CAD build for the part. Positions are in the model's coordinates, mm. Face numbers are marked on the shaded views. A direction names the side the tool comes from. Give positions to 0.01 mm unless a question says otherwise; leave off trailing zeros. Loops run counter-clockwise (first coordinate to the right, second up) from the corner with the lowest first, then second, coordinate; pieces in that order, holes last. Notation, with made-up numbers: M 64,-3.5 L 83,-3.5 A6 ccw 83,4.5 Z; hole C 47,-13 d10. An arc over 180 degrees is marked long. Answer as CSV lines item,"result".
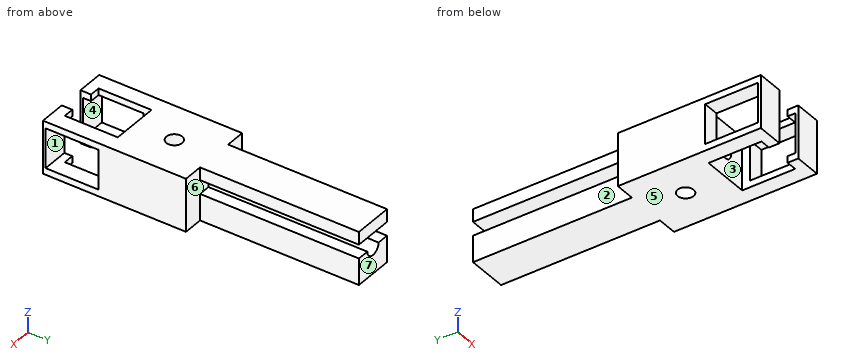
from build123d import *

# Parameters (mm, degrees)
F0_R     = 3.81
F0_W     = 7.62
F0_H     = 25.4
F0_H_2   = 5.08
F0_W_2   = 5.08
F1_DEPTH = 25.4
F2_R     = 3.81
F3_DEPTH = 114.301
F4_W     = 25.4
F4_H     = 19.05
F5_DEPTH = 38.101
F6_W     = 76.2
F6_H     = 6.593191
F7_DEPTH = 28.576


with BuildPart() as f1:
    # F0 (on Top) → F1 (new body)
    with BuildSketch(Plane.XY):
        Polygon((-9.525, 19.05), (-19.05, 19.05), (-19.05, -19.05), (-11.43, -19.05), (11.43, -19.05), (19.05, -19.05), (19.05, 19.05), (9.525, 19.05), (0, 19.05), align=None)
        Circle(F0_R, mode=Mode.SUBTRACT)
        Polygon((-9.525, 95.25), (-9.525, 19.05), (0, 19.05), (9.525, 19.05), (9.525, 95.25), align=None)
        with Locations((-15.24, -31.75)):
            Rectangle(F0_W, F0_H)
        with Locations((-15.24, -46.99)):
            Rectangle(F0_W, F0_H_2)
        with Locations((15.24, -31.75)):
            Rectangle(F0_W, F0_H)
        with Locations((-8.89, -46.99)):
            Rectangle(F0_W_2, F0_H_2)
        with Locations((15.24, -46.99)):
            Rectangle(F0_W, F0_H_2)
        with Locations((8.89, -46.99)):
            Rectangle(F0_W_2, F0_H_2)
    extrude(amount=F1_DEPTH)

    # F2 (on face) → F3 (cut, through all)
    with BuildSketch(Plane.XZ.offset(19.05)):
        with Locations((0, 12.7)):
            Circle(F2_R)
    extrude(amount=-F3_DEPTH, mode=Mode.SUBTRACT)

    # F4 (on face) → F5 (cut, through all)
    with BuildSketch(Plane.YZ.offset(19.05)):
        with Locations((-35.56, 12.7)):
            Rectangle(F4_W, F4_H)
    extrude(amount=-F5_DEPTH, mode=Mode.SUBTRACT)

    # F6 (on face) → F7 (cut, through all)
    with BuildSketch(Plane.YZ.offset(9.525)):
        with Locations((57.15, 15.996595)):
            Rectangle(F6_W, F6_H)
    extrude(amount=-F7_DEPTH, mode=Mode.SUBTRACT)


solid = f1.part
1) Flat gauge pins, fed straight in: pin 1 (7.5 mm diameter, centred on x = -5, z = 18.5, fed in from +Y); pin 2 (6 mm diameter, centred on x = 0, y = 0, fed in from -Z); pin 3 (9 mm diameter, centred on x = 0, z = 12.7, fed in from -Y); pin 4 (6.5 mm diameter, centred on x = -14.5, z = 12.5, fed in from +Y). Where does each tip first touch, or does it go through?
Answer below:
pin 1,"stops at y = 95.25"
pin 2,"passes through"
pin 3,"stops at y = -19.05"
pin 4,"stops at y = 19.05"
2) Which spindle directions (+Z, -Z, +X, -X, +Y, -Y) get a long thin tool onto all of the face, cutting with end or side? Do the marked faces 1, 2 and 3. Say none if no direction does.
Answer below:
face 1,"+X, -X"
face 2,"+Z, -Z, -X, +Y"
face 3,"+Z, -Z"
3) Band-saw the part on D-D on x = 0. Give the cut face in (y, z).
Answer below:
outline,"M -19.05,0 L -3.81,0 L -3.81,8.89 L -19.05,8.89 Z; M -19.05,16.51 L -3.81,16.51 L -3.81,25.4 L -19.05,25.4 Z; M 3.81,0 L 95.25,0 L 95.25,8.89 L 3.81,8.89 Z; M 3.81,16.51 L 19.05,16.51 L 19.05,19.29 L 95.25,19.29 L 95.25,25.4 L 3.81,25.4 Z"
4) Drill centre lines: line 1 (Y direction, x = 0, z = 8.75); line 2 (Z direction, x = -4, y = 71.5); line 3 (Z direction, x = 0, y = 28). Where is each one in solid material? Low to high. Write a range as from..to.
Answer below:
line 1,"y = -19.05..-3.81, 3.81..95.25"
line 2,"z = 0..12.7, 19.29..25.4"
line 3,"z = 0..8.89, 19.29..25.4"
5) Band-saw the part on B-B on z = 17.75. Give the cut face in (x, y).
Answer below:
outline,"M -19.05,-49.53 L -6.35,-49.53 L -6.35,-48.26 L -19.05,-48.26 Z; M -19.05,-22.86 L -11.43,-22.86 L -11.43,-19.05 L 11.43,-19.05 L 11.43,-22.86 L 19.05,-22.86 L 19.05,19.05 L -19.05,19.05 Z; M 6.35,-49.53 L 19.05,-49.53 L 19.05,-48.26 L 6.35,-48.26 Z; hole C 0,0 d7.62"
6) Band-saw the part on C-C on x = -16. Give the cut face in (y, z) (3 decimals), and give its area (3 significant figures).
Answer below:
outline,"M -49.53,0 L 19.05,0 L 19.05,25.4 L -49.53,25.4 Z; hole M -48.26,3.175 L -22.86,3.175 L -22.86,22.225 L -48.26,22.225 Z"
area,"1,260 mm^2"
7) Band-saw the part on A-A on y = 68. Give the cut face in (x, z) (3 decimals), and give its area (3 significant figures).
Answer below:
outline,"M -9.525,0 L 9.525,0 L 9.525,12.7 L 3.81,12.7 A3.81 cw -3.81,12.7 L -9.525,12.7 Z; M -9.525,19.293 L 9.525,19.293 L 9.525,25.4 L -9.525,25.4 Z"
area,"335 mm^2"
8) Mould opens along Z. For the marked faces 4, 5, 6 and 7 say: +Z half, -Z half, draft (parallel to the pull), parting line (faces both ways), or undercut.
Answer below:
face 4,"undercut"
face 5,"-Z half"
face 6,"undercut"
face 7,"draft"
